Autodesk Inventor part; units mm, degrees
ref_plane "YZ Plane" through (0, 0, 0) normal (1, 0, 0) x (0, 1, 0)
ref_plane "XZ Plane" through (0, 0, 0) normal (0, 1, 0) x (-1, 0, 0)
ref_plane "XY Plane" through (0, 0, 0) normal (0, 0, 1) x (1, 0, 0)
sketch "Sketch1" plane through (0, 0, 0) normal (0, 1, 0) x (-1, 0, 0)
  circle A0 centre (0, 0) radius 72.5
  circle A1 centre (0, 0) radius 75
  dimension "d0" = 150
  dimension "d1" = 145
extrude "Extrusion1" add sketch "Sketch1" along normal blind 110
sketch "Sketch2" plane through (0, 0, 0) normal (0, 1, 0) x (-1, 0, 0)
  circle A0 centre (0, 0) radius 40
  circle A1 centre (0, 0) radius 37.5
  dimension "d4" = 75
  dimension "d5" = 2.5
extrude "Extrusion2" add sketch "Sketch2" along normal blind 75
sketch "Sketch3" plane through (0, 0, 0) normal (0, -1, 0) x (1, 0, 0)
  circle A0 centre (0, 0) radius 80
  circle A1 centre (0, 0) radius 40
  dimension "d8" = 160
extrude "Extrusion3" add sketch "Sketch3" along normal blind 2.5
sketch "Sketch4" plane through (0, 0, 0) normal (0, -1, 0) x (1, 0, 0)
  circle A0 centre (0, 0) radius 40
  circle A1 centre (0, 0) radius 37.5
extrude "Extrusion4" add sketch "Sketch4" along normal blind 65
properties part number "_Ref_SkimmerCup"
For this review, take the finished solid that the model builds, in its own axes (mm). A direction names the side the tool comes from. Coordinates: 2 decimals unless noted, no trailing zeros. Loops run counter-clockwise (first coordinate to the right, second up) from the corner with the lowest first, then second, coordinate; pieces in that order, holes last. Notation, with made-up numbers: (72.25, -23) - (115.25, -23) arc R21 ccw to (115.25, 11) - close; hole circle Ø6 at (45, -10). An arc over 180 degrees is marked (long way). Use a Markdown table: item, result. Add a question column.
Item 1: For line 1 (Z direction, x = 0, y = 70); line 2 (Z direction, x = 0, y = -43.5); line 3 (Z direction, x = 0, y = 76), list the stretches that pass through material, from the lowest coordinate up.
Item 2: Mouldability with a two-part tool opening along X and no side actions: class faces 1 (the face through (31, 0, -31)), 2 (the face through (23.3, 0, 71.5)), 3 (the face through (-8.67, -33.31, 39.05)) as pulls with the +X half, pulls with the -X half, needs draft (parallel to the pull), parting line crosses it, or undercut.
Item 3: We need section C-C (y = 19). Give the boundary of the cut face in (x, z).
Item 4: Tool access review of faces 4 (the face through (12, -65, 36)), 5 (the face through (17, -2.5, 37)), 6 (the face through (8.67, 36.98, 39.05)): name each direction out of +Z, -Z, +X, -X, +Y, -Y from which nothing blocks a thin tool from reaching the whole face with its end or side.
Item 5: We need section B-B (x = 0). Give the boundary of the cut face in (y, z), and give its area (3 significant figures).
Item 6: We need section D-D (y = -43). Give the boundary of the cut face in (x, z), and give its area (3 significant figures).
Item 7: We need section A-A (z = 0). Give the boundary of the cut face in (x, y), and give its area (3 significant figures).
Item 8: Insertion check: pin 1 Ø8 at (x, z) = (-31.5, 36) entering from -Y; pin 2 Ø12 at (x, y) = (34.5, 69) entering from -Z; pin 3 Ø8 at (x, y) = (12.5, -45.5) entering from -Z. Each pin has a flat end and moves straight along its axis. Give the tip position at first contact, or say it passes through.
Results list:
| question | item | result |
|---|---|---|
| 1 | line 1 | z = -75 to -72.5, -40 to -37.5, 37.5 to 40, 72.5 to 75 |
| 1 | line 2 | z = -40 to -37.5, 37.5 to 40 |
| 1 | line 3 | z = -75 to -72.5, 72.5 to 75 |
| 2 | face 1 | undercut |
| 2 | face 2 | needs draft |
| 2 | face 3 | parting line crosses it |
| 3 | outline | circle Ø150 at (0, 0); circle Ø80 at (0, 0); hole circle Ø145 at (0, 0); hole circle Ø75 at (0, 0) |
| 4 | face 4 | +Z, -Z, +X, -X, -Y |
| 4 | face 5 | -Y |
| 4 | face 6 | +Y |
| 5 | outline | (-65, -40) - (-2.5, -40) - (-2.5, -80) - (0, -80) - (0, -75) - (110, -75) - (110, -72.5) - (0, -72.5) - (0, -40) - (75, -40) - (75, -37.5) - (-65, -37.5) - close; (-65, 37.5) - (75, 37.5) - (75, 40) - (0, 40) - (0, 72.5) - (110, 72.5) - (110, 75) - (0, 75) - (0, 80) - (-2.5, 80) - (-2.5, 40) - (-65, 40) - close |
| 5 | area | 1,450 mm^2 |
| 6 | outline | circle Ø80 at (0, 0); hole circle Ø75 at (0, 0) |
| 6 | area | 609 mm^2 |
| 7 | outline | (-80, -2.5) - (-40, -2.5) - (-40, -65) - (-37.5, -65) - (-37.5, 75) - (-40, 75) - (-40, 0) - (-72.5, 0) - (-72.5, 110) - (-75, 110) - (-75, 0) - (-80, 0) - close; (37.5, -65) - (40, -65) - (40, -2.5) - (80, -2.5) - (80, 0) - (75, 0) - (75, 110) - (72.5, 110) - (72.5, 0) - (40, 0) - (40, 75) - (37.5, 75) - close |
| 7 | area | 1,450 mm^2 |
| 8 | pin 1 | stops at y = -2.5 |
| 8 | pin 2 | stops at z = -69.37 |
| 8 | pin 3 | stops at z = -39.09 |
